Can you work these out from the model? Positions are in its coordinate system, mm. A direction names the side the tool comes from. Give positions to 0.01 mm unless a question says otherwise; leave off trailing zeros. Write each loop counter-clockwise with the first axis right and the second up, starting at its lowest first coordinate (ties: lowest second). Pieces come first, ordered by that corner, then holes.
1. On a 3-axis mill with a long thin cutter (end or side, diameter ignored), from which of +Z, -Z, +X, -X, +Y, -Y can I reach the whole of each face in a straight line? I mean faces 1 (the flat face through (-28, 78, 17)), 2 (the flat face through (24, 90, 8)), 3 (the flat face through (0, 27, 3)), 4 (the flat face through (-26, 37, 15)). Say none if no direction works.
2. Thinking about a two-plate mould opening in Y: for faces 5 (the cylindrical face through (-24.29, -6.35, 8.03)), 6 (the cylindrical face through (-20.86, 36.76, 14.1)), 7 (the cylindrical face through (29.014, 84.309, 21.465)), 8 (the flat face through (-24, 90, 8)), which applies, pulls with the +Y half, pulls with the -Y half, needs draft (parallel to the pull), parting line crosses it, or undercut?
3. If I drill on probe 1 along X at (y, z) = (9.5, 9); probe 2 along X at (y, z) = (84, 16.5); probe 3 along Z at (x, y) = (27, 17.5), over which ranges is the centre line in solid material (lowest first)?
4. Suppose I cut it at C-C (y = 50). Please give me the cut outline in (x, z).
5. I'm going to push flat-ended pins straight in: pin 1 (2 mm diameter, centred on x = -12.5, y = 34.5, fed in from +Z); pin 2 (5.5 mm diameter, centred on x = -26, y = 35, fed in from +Z); pin 3 (5 mm diameter, centred on x = 2, z = 4, fed in from +Y). Where does each tip first touch, or does it pass through?
6. Suppose I cut it at B-B (z = 7.5). Give the number of separate pieces and of enclosed holes in the cut face, and give its area (3 significant figures).
7. Suppose I cut it at D-D (z = 17). Please give me the cut outline in (x, y).
8. Suppose I cut it at A-A (y = 76.5). Please give me the cut outline in (x, z), and give its area (3 significant figures).
```python
from build123d import *

# Parameters (mm, degrees)
F2_DEPTH       = 100
F2_DEPTH_BACK  = 20
F1_R           = 1
F4_DEPTH       = 15
F4_DEPTH_BACK  = 90
F6_R           = 16
F7_DEPTH       = 2
F8_R           = 16
F9_DEPTH       = 2
F11_DEPTH      = 10
F12_R          = 1.2
F13_DEPTH      = 124.25
F13_DEPTH_BACK = 109.5
F14_W          = 125.272244215
F14_H          = 20.9059882909
F15_DEPTH      = 40


with BuildPart() as f2:
    # F1 (on face) → F2 (new body, two sides)
    with BuildSketch(Plane(origin=(0, 0, 0), x_dir=(1, 0, 0), z_dir=(0, -0.7071067812, 0.7071067812))) as f2_sk:
        with BuildLine():
            ThreePointArc((25.13, 0), (24.13, 1), (23.13, 0))
            ThreePointArc((23.13, 0), (24.13, -1), (25.13, 0))
        make_face()
    extrude(amount=F2_DEPTH)
    extrude(f2_sk.sketch, amount=-F2_DEPTH_BACK)



with BuildPart() as f2b:
    # F1 (on face) → F2, piece 2 (new body, two sides)
    with BuildSketch(Plane(origin=(0, 0, 0), x_dir=(1, 0, 0), z_dir=(0, -0.7071067812, 0.7071067812))) as f2_2_sk:
        with Locations((-24.13, 0)):
            Circle(F1_R)
    extrude(amount=F2_DEPTH)
    extrude(f2_2_sk.sketch, amount=-F2_DEPTH_BACK)


with BuildPart() as f2_1:
    add(f2.part)

    add(f2b.part)  # F4 merges F2b
    # F3 (on Front) → F4 (join, two sides)
    with BuildSketch(Plane.XZ) as f4_sk:
        with BuildLine():
            Line((-30, 15), (-30, 0))
            Line((-30, 0), (30, 0))
            Line((30, 0), (30, 15))
            Line((30, 15), (23, 15))
            ThreePointArc((23, 15), (20.8786796564, 14.1213203436), (20, 12))
            Line((20, 12), (20, 3))
            Line((20, 3), (-20, 3))
            Line((-20, 3), (-20, 12))
            ThreePointArc((-20, 12), (-20.8786796564, 14.1213203436), (-23, 15))
            Line((-23, 15), (-30, 15))
        make_face()
    extrude(amount=F4_DEPTH)
    extrude(f4_sk.sketch, amount=-F4_DEPTH_BACK)

    # F6 (on face) → F7 (join)
    with BuildSketch(Plane(origin=(-30, 0, 0), x_dir=(0, -1, 0), z_dir=(-1, 0, 0))):
        with Locations((-76.5, 7.5)):
            Circle(F6_R)
    extrude(amount=-F7_DEPTH)

    # F8 (on face) → F9 (join)
    with BuildSketch(Plane.YZ.offset(30)):
        with Locations((76.5, 7.5)):
            Circle(F8_R)
    extrude(amount=-F9_DEPTH)

    # F10 (on Top) → F11 (cut)
    with BuildSketch(Plane.XY):
        Polygon((20, 90), (-20, 90), (-20, 77.4333529874), (-20, 70), (20, 70), align=None)
    extrude(amount=F11_DEPTH, mode=Mode.SUBTRACT)

    # F12 (on face) → F13 (cut, two sides)
    with BuildSketch(Plane(origin=(0, 0, 0), x_dir=(1, 0, 0), z_dir=(0, -0.7071067812, 0.7071067812))) as f13_sk:
        with BuildLine():
            ThreePointArc((25.33, 0), (24.13, 1.2), (22.93, 0))
            ThreePointArc((22.93, 0), (24.13, -1.2), (25.33, 0))
        make_face()
        with Locations((-24.13, 0)):
            Circle(F12_R)
    extrude(amount=F13_DEPTH, mode=Mode.SUBTRACT)
    extrude(f13_sk.sketch, amount=-F13_DEPTH_BACK, mode=Mode.SUBTRACT)

    # F14 (on Right) → F15 (cut, symmetric)
    with BuildSketch(Plane.YZ):
        with Locations((62.6361221075, -10.4529941455)):
            Rectangle(F14_W, F14_H)
    extrude(amount=F15_DEPTH, both=True, mode=Mode.SUBTRACT)


solid = f2_1.part
```
Checks:
1. face 1: +Z, +Y
1. face 2: +Z, -Z, +Y
1. face 3: +Z, +Y, -Y
1. face 4: +Z, -Y
2. face 5: undercut
2. face 6: needs draft
2. face 7: parting line crosses it
2. face 8: pulls with the +Y half
3. probe 1: x = -30 to -20, 20 to 30
3. probe 2: x = -30 to -28, 28 to 30
3. probe 3: z = 0 to 15
4. outline: (-30, 0) - (30, 0) - (30, 15) - (23, 15) arc R3 ccw to (20, 12) - (20, 3) - (-20, 3) - (-20, 12) arc R3 ccw to (-23, 15) - (-30, 15) - close
5. pin 1: stops at z = 3
5. pin 2: stops at z = 15
5. pin 3: stops at y = 70
6. separate pieces: 2
6. enclosed holes: 2
6. area: 2,100 mm2
7. outline: (-30, 63.63) - (-28, 63.63) - (-28, 89.37) - (-30, 89.37) - close; (28, 63.63) - (30, 63.63) - (30, 89.37) - (28, 89.37) - close
8. outline: (-30, 0) - (-20, 0) - (-20, 12) arc R3 ccw to (-23, 15) - (-28, 15) - (-28, 23.5) - (-30, 23.5) - close; (20, 0) - (30, 0) - (30, 23.5) - (28, 23.5) - (28, 15) - (23, 15) arc R3 ccw to (20, 12) - close
8. area: 330 mm2
